Part model, mm, in its own coordinate system. Face numbers are marked on the shaded views. A direction names the side the tool comes from. Give positions to 0.01 mm unless a question says otherwise; leave off trailing zeros. Write each loop counter-clockwise with the first axis right and the second up, starting at its lowest first coordinate (ties: lowest second). Pieces come first, ordered by that corner, then holes.
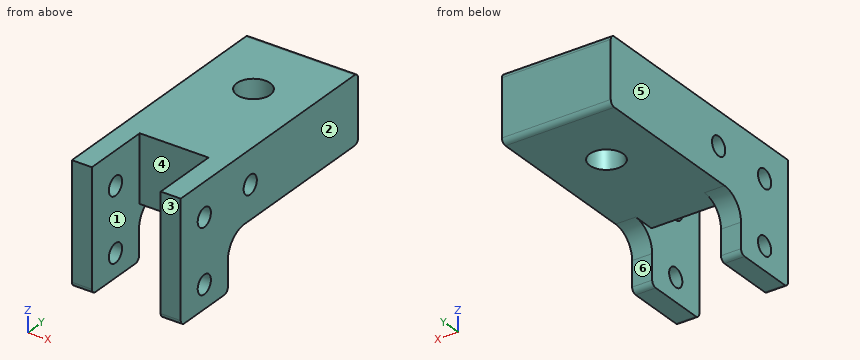
from build123d import *

# Parameters (mm, degrees)
EXTRUDE1_DEPTH      = 10.3
EXTRUDE1_DEPTH_BACK = 10.3
SKETCH1_W           = 20
SKETCH1_H           = 55
EXTRUDE2_DEPTH      = 6
SKETCH4_R           = 2.8
EXTRUDE3_DEPTH      = 78.478061411
SKETCH5_R           = 5
EXTRUDE4_DEPTH      = 77.326797391
FILLET2_R           = 1.5
SKETCH_1_W          = 32.6
SKETCH_1_H          = 73.8
CUT_EXTRUDE_1_DEPTH = 77.326797391


with BuildPart() as part:
    # Sketch1 → Extrude1 (new, two sides: drawn at the far end of the back side and taken through both)
    with BuildSketch(Plane(origin=(0, 0, 0), x_dir=(0, 0, -1), z_dir=(1, 0, 0)).offset(-EXTRUDE1_DEPTH_BACK)):
        with Locations((0, 37.8)):
            Rectangle(SKETCH1_W, SKETCH1_H)
    extrude(amount=EXTRUDE1_DEPTH + EXTRUDE1_DEPTH_BACK)

    # Sketch2 → Extrude2 (add)
    with BuildSketch(Plane(origin=(10.3, 0, 0), x_dir=(0, 0, -1), z_dir=(1, 0, 0))):
        with BuildLine():
            Line((26, 10), (17, 10))
            ThreePointArc((17, 10), (12.050252532, 12.050252532), (10, 17))
            Line((10, 17), (10, 65.3))
            Line((10, 65.3), (-10, 65.3))
            Line((-10, 65.3), (-10, 17))
            ThreePointArc((-10, 17), (-12.050252532, 12.050252532), (-17, 10))
            Line((-17, 10), (-26, 10))
            Line((-26, 10), (-26, -10))
            Line((-26, -10), (26, -10))
            Line((26, -10), (26, 10))
        make_face()
    extrude2 = extrude(amount=EXTRUDE2_DEPTH)

    # Mirror2: Extrude2 across plane
    add(extrude2.mirror(Plane(origin=(0, 0, 0), x_dir=(0, 0, 1), z_dir=(1, 0, 0))))

    # Sketch4 → Extrude3 (cut, through all)
    with BuildSketch(Plane(origin=(16.3, 0, 0), x_dir=(0, 0, -1), z_dir=(1, 0, 0))):
        Circle(SKETCH4_R)
        with Locations((19, 0)):
            Circle(SKETCH4_R)
        with Locations((-19, 0)):
            Circle(SKETCH4_R)
        with Locations((0, 19.5)):
            Circle(SKETCH4_R)
    extrude(amount=-EXTRUDE3_DEPTH, mode=Mode.SUBTRACT)

    # Sketch5 → Extrude4 (cut, through all)
    with BuildSketch(Plane.XY.offset(10)):
        with Locations((0, 44)):
            Circle(SKETCH5_R)
    extrude(amount=-EXTRUDE4_DEPTH, mode=Mode.SUBTRACT)

    # Fillet2
    fillet2_edges = [part.edges().sort_by_distance(p)[0] for p in [
        (13.3, 10, 26),
        (13.3, -10, 26),
        (13.3, -10, -26),
        (13.3, 10, -26),
        (-13.3, -10, 26),
        (-13.3, 10, 26),
        (-13.3, 10, -26),
        (-13.3, -10, -26),
        (0, 65.3, 10),
        (0, 65.3, -10),
    ]]
    fillet(fillet2_edges, radius=FILLET2_R)

    # Эскиз1 → Вырез-Вытянуть1 (cut, through all)
    with BuildSketch(Plane(origin=(0, 0, 10), x_dir=(-1, 0, 0), z_dir=(0, 0, -1))):
        with Locations((0, 26.9)):
            Rectangle(SKETCH_1_W, SKETCH_1_H)
    extrude(amount=-CUT_EXTRUDE_1_DEPTH, mode=Mode.SUBTRACT)


solid = part.part
1) 3-axis set-ups, long thin cutter, end or side, ignore diameter. For the marked faces 5 and 6: which of +Z, -Z, +X, -X, +Y, -Y reach the whole face in a straight line?
Check result:
face 5: +Z, -Z, -X, +Y, -Y
face 6: -Z, +X, -X, +Y
2) Saw through at A-A (z = 0). Write the cut outline in (x, y).
Check result:
outline: (-16.3, -10) - (-10.3, -10) - (-10.3, -2.8) - (-16.3, -2.8) - close; (-16.3, 2.8) - (-10.3, 2.8) - (-10.3, 10.3) - (10.3, 10.3) - (10.3, 2.8) - (16.3, 2.8) - (16.3, 16.7) - (-16.3, 16.7) - close; (-16.3, 22.3) - (16.3, 22.3) - (16.3, 65.3) - (-16.3, 65.3) - close; (10.3, -10) - (16.3, -10) - (16.3, -2.8) - (10.3, -2.8) - close; hole circle Ø10 at (0, 44)
3) Drill centre lines: L1, parallel to X at y = -3.5, z = -8; L2, parallel to Z at x = 2, y = 38.5; L3, parallel to Y at x = -13, z = -19. Where is each one in solid material? Low to high.
Check result:
L1: x = -16.3 to -10.3, 10.3 to 16.3
L2: z = -10 to 10
L3: y = -10 to -2.8, 2.8 to 10
4) Mould opens along X. For the marked faces 1, 2, 3 and 4 say: +X half, -X half, draft (parallel to the pull), parting line (faces both ways), or undercut.
Check result:
face 1: undercut
face 2: +X half
face 3: draft
face 4: undercut
5) Flat gauge pins, fed straight in: P1, Ø10, axis at x = 0.5, y = 30.5, coming from the -Z side; P2, Ø8, axis at x = 9.5, y = 10, coming from the -Z side; P3, Ø4.5, axis at y = 0, z = 0, coming from the -X side; P4, Ø3, axis at x = -13.5, z = -22, coming from the +Y side. Where does each tip first touch, or does it go through?
Check result:
P1: stops at z = -10
P2: stops at z = -26
P3: passes through
P4: stops at y = 10
6) Saw through at D-D (x = 0). Write the cut outline in (y, z).
Check result:
outline: (10.3, -10) - (39, -10) - (39, 10) - (10.3, 10) - close; (49, -10) - (63.8, -10) arc R1.5 ccw to (65.3, -8.5) - (65.3, 8.5) arc R1.5 ccw to (63.8, 10) - (49, 10) - close; hole circle Ø5.6 at (19.5, 0)
7) Saw through at B-B (x = -7). Write the cut outline in (y, z), and give its area (3 significant figures).
Check result:
outline: (10.3, -10) - (63.8, -10) arc R1.5 ccw to (65.3, -8.5) - (65.3, 8.5) arc R1.5 ccw to (63.8, 10) - (10.3, 10) - close; hole circle Ø5.6 at (19.5, 0)
area: 1,070 mm2
8) Saw through at C-C (y = 19.5). Write the cut outline in (x, z).
Check result:
outline: (-16.3, -10) - (16.3, -10) - (16.3, -2.8) - (-16.3, -2.8) - close; (-16.3, 2.8) - (16.3, 2.8) - (16.3, 10) - (-16.3, 10) - close
